from build123d import *

# Parameters (mm, degrees)
SKETCH1_R           = 2.25
BOSS_EXTRUDE1_DEPTH = 5
SKETCH2_W           = 53
SKETCH2_H           = 5.069282957
BOSS_EXTRUDE2_DEPTH = 38
BOSS_EXTRUDE3_DEPTH = 5
BOSS_EXTRUDE4_DEPTH = 5
SKETCH5_R           = 11.25
SKETCH5_R_2         = 2
CUT_EXTRUDE1_DEPTH  = 49


with BuildPart() as part:
    # Sketch1 → Boss-Extrude1 (new body)
    with BuildSketch(Plane.XY):
        Polygon((0, 0), (0, 43), (43, 43), (43, 0), (59, 0), (59, 48), (-16, 48), (-16, 0), align=None)
        with Locations((-10, 40)):
            Circle(SKETCH1_R, mode=Mode.SUBTRACT)
        with Locations((53, 40)):
            Circle(SKETCH1_R, mode=Mode.SUBTRACT)
        with Locations((53, 8)):
            Circle(SKETCH1_R, mode=Mode.SUBTRACT)
        with Locations((-10, 8)):
            Circle(SKETCH1_R, mode=Mode.SUBTRACT)
    extrude(amount=BOSS_EXTRUDE1_DEPTH)

    # Sketch2 → Boss-Extrude2 (add)
    with BuildSketch(Plane.XY.offset(5)):
        with Locations((21.5, 45.465358522)):
            Rectangle(SKETCH2_W, SKETCH2_H)
    extrude(amount=BOSS_EXTRUDE2_DEPTH)

    # Sketch3 → Boss-Extrude3 (add)
    with BuildSketch(Plane.ZY.offset(5)):
        Polygon((5, 48), (5, 0), (43, 42.930717043), (43, 48), align=None)
    extrude(amount=-BOSS_EXTRUDE3_DEPTH)

    # Sketch4 → Boss-Extrude4 (add)
    with BuildSketch(Plane(origin=(48, 0, 0), x_dir=(0, 0, -1), z_dir=(1, 0, 0))):
        Polygon((-43, 48), (-43, 42.930717043), (-5, 0), (-5, 48), align=None)
    extrude(amount=-BOSS_EXTRUDE4_DEPTH)

    # Sketch5 → Cut-Extrude1 (cut, through all)
    with BuildSketch(Plane(origin=(0, 48, 0), x_dir=(1, 0, 0), z_dir=(0, 1, 0))):
        with Locations((21.5, -21.5)):
            Circle(SKETCH5_R)
        with Locations((5.98, -5.98)):
            Circle(SKETCH5_R_2)
        with Locations((37.02, -5.98)):
            Circle(SKETCH5_R_2)
        with Locations((37.02, -37.02)):
            Circle(SKETCH5_R_2)
        with Locations((5.98, -37.02)):
            Circle(SKETCH5_R_2)
    extrude(amount=-CUT_EXTRUDE1_DEPTH, mode=Mode.SUBTRACT)


solid = part.part
Source: CAD feature listing. Evaluate the final solid. Frame: model axes, mm. A direction names the side the tool comes from. Give positions to 0.01 mm unless a question says otherwise; leave off trailing zeros. Write each loop counter-clockwise with the first axis right and the second up, starting at its lowest first coordinate (ties: lowest second). Pieces come first, ordered by that corner, then holes. Notation, with made-up numbers: M 14.25,-39 L 47.25,-39 A19 cw 47.25,-33 Z; hole C 28.25,76 d5. An arc over 180 degrees is marked long. Return JSON: item names as keys, results as strings. Group by question number.
1) Cut plane B-B, the plane z = 15.5. Output: boundary loops of the cut face in (x, y), plus the area to 3 significant figures.
2) Cut plane D-D, the plane z = 7. Output: boundary loops of the cut face in (x, y).
3) Cut plane A-A, the plane x = 53. Output: boundary loops of the cut face in (y, z), plus the area to 3 significant figures.
4) Cut plane C-C, the plane y = 8. Output: boundary loops of the cut face in (x, z), plus the area to 3 significant figures.
5) Pin query (flat end, axial travel): P1, Ø19, axis at x = 18.5, z = 22.5, coming from the -Y side; P2, Ø21.5, axis at y = 18.5, z = 31.5, coming from the +X side; P3, Ø12, axis at x = -11.5, y = 12.5, coming from the +Z side; P4, Ø4, axis at y = 13, z = 19.5, coming from the +X side. Return the tip coordinate at first contact, or that it passes through.
6) Pull-direction query (Y, two-part tool) for faces 6 (the face through (51.34, 41.52, 2.46)), 7 (the face through (-8, 0, 2)), 8 (the face through (13, 48, 12)), 9 (the face through (53, 24, 5)); classes: pulls with the +Y half, pulls with the -Y half, needs draft (parallel to the pull), parting line crosses it, or undercut.
7) Set-up query: faces 1 (the face through (16, 42.931, 32)), 2 (the face through (51, 0, 2)), 3 (the face through (-5, 29, 20)), 4 (the face through (21, 43, 2)), 5 (the face through (36.586, 45.501, 38.972)). Return all of +Z, -Z, +X, -X, +Y, -Y with unobstructed straight access to the full face (end or side cutting, diameter ignored); none if empty.
8) Material intervals for line 1 along Y through (x, z) = (-10, 3.5); line 2 along X through (y, z) = (3, 5.5); line 3 along Z through (x, y) = (5.98, 46.7), sorted ascending. Write a range as [from, to].
Recorded:
{
 "1": {"outline": "M -5,11.86 L 0,11.86 L 0,42.93 L 11.98,42.93 L 11.98,48 L -5,48 Z; M 31.02,42.93 L 43,42.93 L 43,11.86 L 48,11.86 L 48,48 L 31.02,48 Z", "area": "483 mm²"},
 "2": {"outline": "M -5,2.26 L 0,2.26 L 0,42.93 L 4.26,42.93 L 4.26,48 L -5,48 Z; M 7.7,42.93 L 35.3,42.93 L 35.3,48 L 7.7,48 Z; M 38.74,42.93 L 43,42.93 L 43,2.26 L 48,2.26 L 48,48 L 38.74,48 Z"},
 "3": {"outline": "M 0,0 L 5.75,0 L 5.75,5 L 0,5 Z; M 10.25,0 L 37.75,0 L 37.75,5 L 10.25,5 Z; M 42.25,0 L 48,0 L 48,5 L 42.25,5 Z", "area": "195 mm²"},
 "4": {"outline": "M -16,0 L -12.25,0 L -12.25,5 L -16,5 Z; M -7.75,0 L 0,0 L 0,12.08 L -5,12.08 L -5,5 L -7.75,5 Z; M 43,0 L 50.75,0 L 50.75,5 L 48,5 L 48,12.08 L 43,12.08 Z; M 55.25,0 L 59,0 L 59,5 L 55.25,5 Z", "area": "186 mm²"},
 "5": {"P1": "stops at y = 42.93", "P2": "stops at x = 48", "P3": "stops at z = 5", "P4": "passes through"},
 "6": {"face 6": "undercut", "face 7": "pulls with the -Y half", "face 8": "pulls with the +Y half", "face 9": "needs draft"},
 "7": {"face 1": "+Z, -Z, -Y", "face 2": "+Z, -Z, +X, -X, -Y", "face 3": "+Z, -X, +Y, -Y", "face 4": "-Z, -Y", "face 5": "+Y, -Y"},
 "8": {"line 1": "y = [0, 5.75], [10.25, 37.75], [42.25, 48]", "line 2": "x = [-5, 0], [43, 48]", "line 3": "z = [0, 3.98], [7.98, 35.02], [39.02, 43]"}
}
